Design review of the part shown in the three views and the two pictorial views. Dimensions are in mm from the part's minimum x, y and z. Coordinates: 2 decimals unless noted, no trailing zeros. Loops run counter-clockwise (first coordinate to the right, second up) from the corner with the lowest first, then second, coordinate; pieces in that order, holes last.
Q1. For P1, Ø1.2, axis at x = 2, y = 2.5, coming from the -Z side; P2, Ø1.5, axis at x = 70.5, y = 2, coming from the +Z side (1 decimal); P3, Ø1.2, axis at y = 1, z = 4, coming from the -X side, all flat-tipped, find the tip position at first contact; note any pin that passes through.
Q2. Add section A-A on x = 75. Give the boundary of the cut face in (y, z) (1 decimal).
Q3. Wall thickness on probe 1 along X at (y, z) = (3, 107.5) (1 decimal); probe 2 along Z at (x, y) = (75, 2.9) (1 decimal); probe 3 along Z at (x, y) = (78.5, 0.35) (1 decimal): over which ranges is each line inside the solid? List them lowest first.
Q4. Add section B-B on y = 0.65. Give the number of separate pieces and of enclosed holes in the cut face, and give its area (3 significant figures).
Q5. Add section D-D on z = 182. Give the boundary of the cut face in (x, y).
Q6. Add section C-C on x = 32.5. Give the boundary of the cut face in (y, z) (1 decimal).
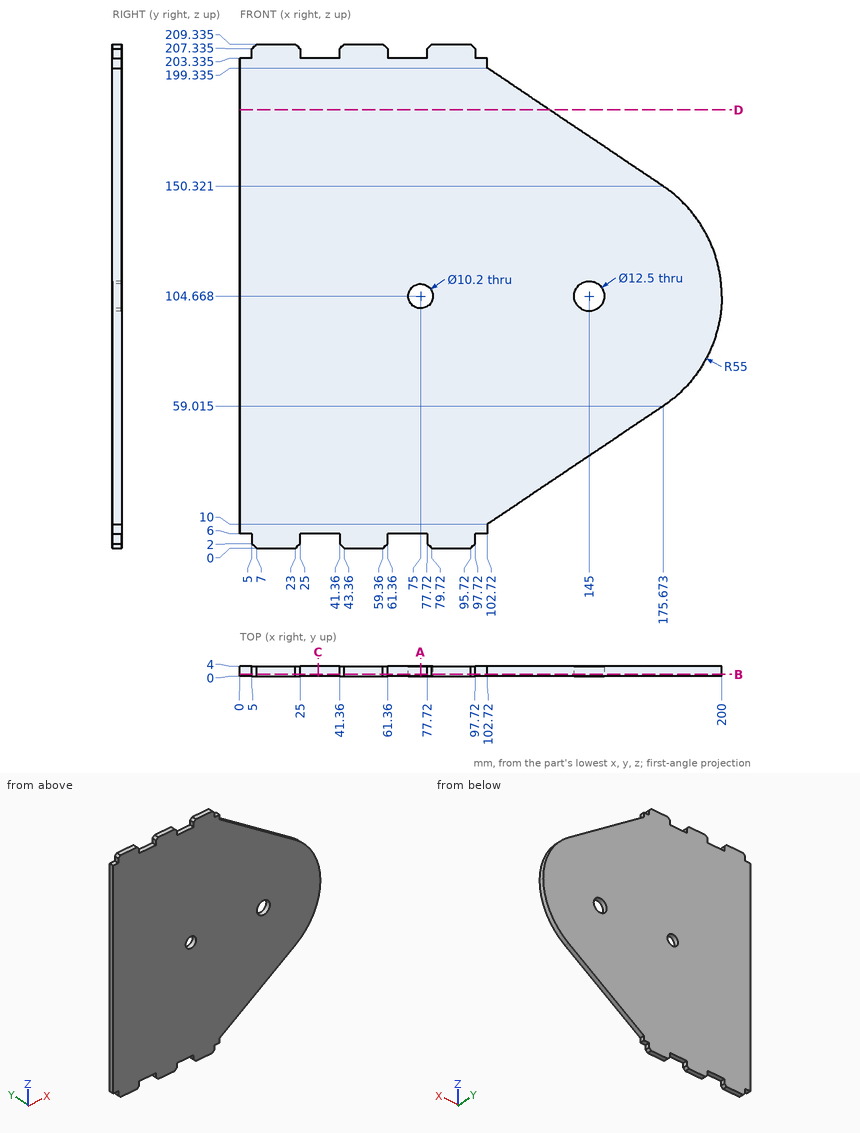
Entries:
1. P1: stops at z = 6
1. P2: stops at z = 203.3
1. P3: stops at x = 5
2. outline: (0, 6) - (4, 6) - (4, 99.6) - (0, 99.6) - close; (0, 109.8) - (4, 109.8) - (4, 203.3) - (0, 203.3) - close
3. probe 1: x = 0 to 70.8, 79.2 to 139.4, 150.6 to 199.9
3. probe 2: z = 6 to 99.6, 109.8 to 203.3
3. probe 3: z = 1.2 to 101, 108.4 to 208.1
4. separate pieces: 1
4. enclosed holes: 2
4. area: 32,600 mm2
5. outline: (0, 0) - (128.52, 0) - (128.52, 4) - (0, 4) - close
6. outline: (0, 6) - (4, 6) - (4, 203.3) - (0, 203.3) - close
